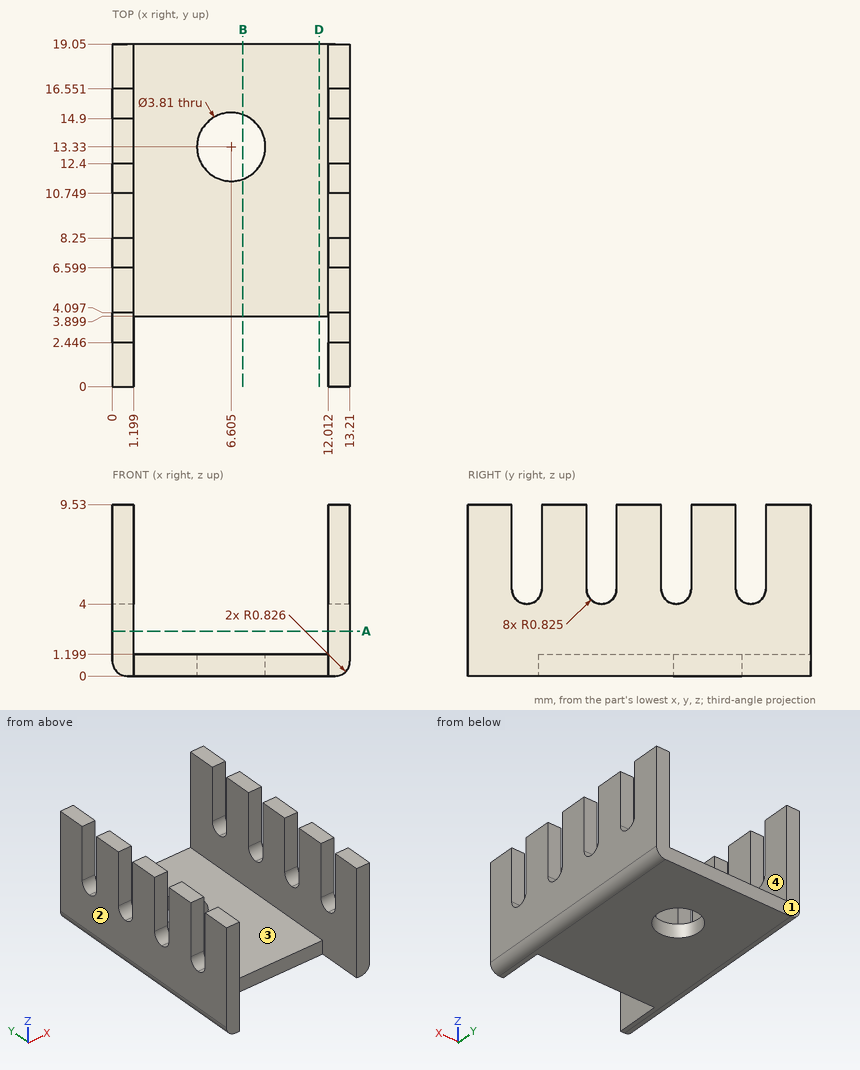
Study the drawing (mm; zero at the part's minimum x, y, z) and answer. Coordinates: 2 decimals unless noted, no trailing zeros. Write each loop counter-clockwise with the first axis right and the second up, starting at its lowest first coordinate (ties: lowest second). Pieces come first, ordered by that corner, then holes. Notation, with made-up numbers: (11.5, 19.5) - (27.5, 19.5) arc R31 ccw to (27.5, 56.5) - close; hole circle Ø2 at (-13.5, -0.75). An arc over 180 degrees is marked (long way). Put each result on its own line as item: value.
1. A flat-ended cylindrical pin translates along its axis: pin 1 Ø2 at (x, y) = (8, 4) entering from +Z. Find the tip coordinate at first contact, or state that the pin passes through.
Answer sheet:
pin 1: stops at z = 1.2
2. Find the intervals of material crossed by line 1 along X through (y, z) = (17.5, 5); line 2 along Z through (x, y) = (2.75, 8), in increasing order. Write a range as from..to.
Answer sheet:
line 1: x = 0..1.2, 12.01..13.21
line 2: z = 0..1.2
3. The part is cut by section A-A on z = 2.5. Give the vertices of the cut face in (x, y).
Answer sheet:
outline: (0, 0) - (1.2, 0) - (1.2, 19.05) - (0, 19.05) - close; (12.01, 0) - (13.21, 0) - (13.21, 19.05) - (12.01, 19.05) - close
4. The part is cut by section B-B on x = 7.25. Give the vertices of the cut face in (y, z).
Answer sheet:
outline: (3.9, 0) - (11.54, 0) - (11.54, 1.2) - (3.9, 1.2) - close; (15.12, 0) - (19.05, 0) - (19.05, 1.2) - (15.12, 1.2) - close
5. The part is cut by section D-D on x = 11.5. Give the vertices of the cut face in (y, z).
Answer sheet:
outline: (3.9, 0) - (19.05, 0) - (19.05, 1.2) - (3.9, 1.2) - close
6. Determine the mould class of the marked faces 1, 2, 3 and 4 for opening direction X: pulls with the +X half, pulls with the -X half, needs draft (parallel to the pull), parting line crosses it, or undercut.
Answer sheet:
face 1: needs draft
face 2: pulls with the -X half
face 3: undercut
face 4: undercut
